Geometry: final body of the model. Coordinates: model frame, mm. Coordinates: 2 decimals unless noted, no trailing zeros. Loops run counter-clockwise (first coordinate to the right, second up) from the corner with the lowest first, then second, coordinate; pieces in that order, holes last. Notation, with made-up numbers: (-29.75, 84) - (11.25, 84) arc R14 cw to (11.25, 106) - close; hole circle Ø10 at (75.25, 27). An arc over 180 degrees is marked (long way). Answer in a Markdown table with one row per item.
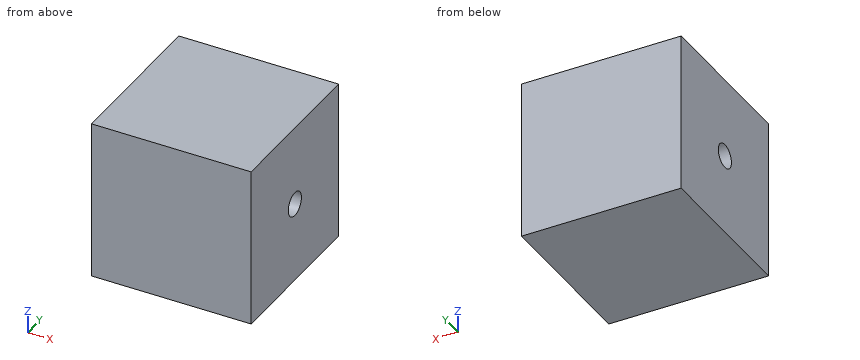
from build123d import *

# Parameters (mm, degrees)
SKETCH1_W           = 20
SKETCH1_H           = 20
BOSS_EXTRUDE1_DEPTH = 20
SKETCH3_R           = 1.5
CUT_EXTRUDE1_DEPTH  = 20


with BuildPart() as part:
    # Sketch1 → Boss-Extrude1 (new body)
    with BuildSketch(Plane(origin=(0, 0, 0), x_dir=(1, 0, 0), z_dir=(0, 1, 0))):
        Rectangle(SKETCH1_W, SKETCH1_H)
    extrude(amount=BOSS_EXTRUDE1_DEPTH)

    # Sketch3 → Cut-Extrude1 (cut)
    with BuildSketch(Plane.ZY.offset(10)):
        with Locations((0, 10)):
            Circle(SKETCH3_R)
    extrude(amount=-CUT_EXTRUDE1_DEPTH, mode=Mode.SUBTRACT)


solid = part.part
(1) Cut plane C-C on x = 4.75. Output: boundary loops of the cut face in (y, z), then the cut area to 3 significant figures.
Verdict:
| item | result |
|---|---|
| outline | (0, -10) - (20, -10) - (20, 10) - (0, 10) - close; hole circle Ø3 at (10, 0) |
| area | 393 mm² |
(2) Cut plane A-A on y = 10. Output: boundary loops of the cut face in (x, z), then the cut area to 3 significant figures.
Verdict:
| item | result |
|---|---|
| outline | (-10, -10) - (10, -10) - (10, -1.5) - (-10, -1.5) - close; (-10, 1.5) - (10, 1.5) - (10, 10) - (-10, 10) - close |
| area | 340 mm² |
(3) Cut plane B-B on z = 0. Output: boundary loops of the cut face in (x, y).
Verdict:
| item | result |
|---|---|
| outline | (-10, 0) - (10, 0) - (10, 8.5) - (-10, 8.5) - close; (-10, 11.5) - (10, 11.5) - (10, 20) - (-10, 20) - close |
(4) Ray query, probe 1 along Y at (x, z) = (2.75, 0); probe 2 along Z at (x, y) = (-6.75, 10.5); probe 3 along Z at (x, y) = (1.5, 10.25). Return the intervals inside material, ascending.
Verdict:
| item | result |
|---|---|
| probe 1 | y = 0 to 8.5, 11.5 to 20 |
| probe 2 | z = -10 to -1.41, 1.41 to 10 |
| probe 3 | z = -10 to -1.48, 1.48 to 10 |
